```python
from build123d import *

# Parameters (mm, degrees)
SKETCH_1_R          = 27.5
SKETCH_1_R_2        = 21.5
SKETCH_1_R_3        = 1.1
EXTRUDE_1_DEPTH     = 5
CUT_EXTRUDE_1_DEPTH = 5
FILLET_1_R          = 1.5


with BuildPart() as part:
    # 草图1 → 凸台-拉伸1 (new body)
    with BuildSketch(Plane(origin=(0, 0, 0), x_dir=(1, 0, 0), z_dir=(0, 1, 0))):
        with Locations(Location((0, 0, 0), (0, 0, 270))):
            Circle(SKETCH_1_R)
        with Locations(Location((0, 0, 0), (0, 0, 270))):
            Circle(SKETCH_1_R_2, mode=Mode.SUBTRACT)
        with Locations(Location((0, 24.5, 0), (0, 0, 270))):
            Circle(SKETCH_1_R_3, mode=Mode.SUBTRACT)
        with Locations(Location((21.217622393, -12.25, 0), (0, 0, 270))):
            Circle(SKETCH_1_R_3, mode=Mode.SUBTRACT)
        with Locations(Location((-21.217622393, -12.25, 0), (0, 0, 270))):
            Circle(SKETCH_1_R_3, mode=Mode.SUBTRACT)
    extrude(amount=EXTRUDE_1_DEPTH)

    # 草图2 → 切除-拉伸1 (cut)
    with BuildSketch(Plane.XZ):
        with BuildLine():
            Line((-2.453357197, -21.359565503), (-4.550320626, -27.120925172))
            ThreePointArc((-4.550320626, -27.120925172), (-20.900792824, -17.871957345), (-27.498537849, -0.283577443))
            Line((-27.498537849, -0.283577443), (-21.481435012, 0.89328037))
            ThreePointArc((-21.481435012, 0.89328037), (-16.340619844, -13.972621197), (-2.453357197, -21.359565503))
        make_face()
    extrude(amount=-CUT_EXTRUDE_1_DEPTH, mode=Mode.SUBTRACT)

    # 圆角1
    fillet_1_edges = [part.edges().sort_by_distance(p)[0] for p in [
        (-21.481435012, 2.5, 0.89328037),
        (-2.453357197, 2.5, -21.359565503),
        (-4.550320626, 2.5, -27.120925172),
        (-27.498537849, 2.5, -0.283577443),
    ]]
    fillet(fillet_1_edges, radius=FILLET_1_R)


solid = part.part
```
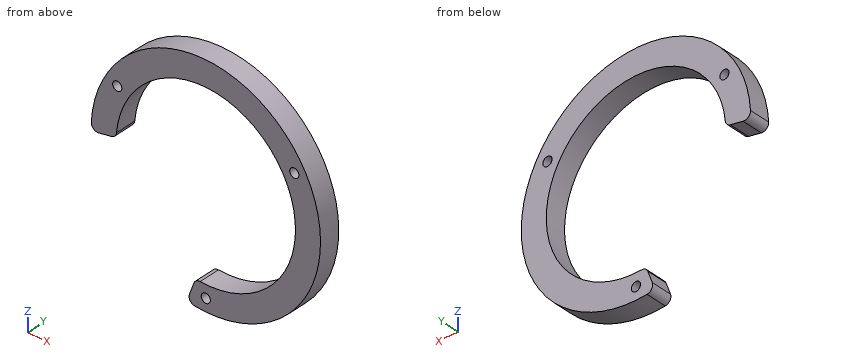
Read the model definition and answer for the solid it produces. Units are mm, in the model's axes. Coordinates: 2 decimals unless noted, no trailing zeros. Write each loop counter-clockwise with the first axis right and the second up, starting at its lowest first coordinate (ties: lowest second). Pieces come first, ordered by that corner, then holes. Notation, with made-up numbers: (72, 62.25) -> (86, 62.25) arc R16 cw to (86, 93.25) -> close; hole circle Ø2 at (57.25, 60.25). An arc over 180 degrees is marked (long way). Write item = value, one per line.
(1) Straight lines are drawn through the part: L1, parallel to X at y = 2.45, z = 12.25; L2, parallel to X at y = 4.45, z = -24.5; L3, parallel to X at y = 1.8, z = 2. For each, find the intervals that lie inside material, in ascending order. Write a range as from..to.
From the geometry:
L1 = -24.62..-22.32, -20.12..-17.67, 17.67..20.12, 22.32..24.62
L2 = -3.6..-1.1, 1.1..12.49
L3 = -27.43..-21.41, 21.41..27.43
(2) Section C-C on y = 1.85 is taken. Write down the section's boundary in (x, z), plus the area to 3 significant figures.
From the geometry:
outline = (-27.45, 1.64) arc R1.5 ccw to (-25.67, 0.07) -> (-22.61, 0.67) arc R1.5 ccw to (-21.41, 2) arc R21.5 cw (long way) to (-1.34, -21.46) arc R1.5 ccw to (-2.85, -22.44) -> (-3.91, -25.37) arc R1.5 ccw to (-2.65, -27.37) arc R27.5 ccw (long way) to start; hole circle Ø2.2 at (-21.22, 12.25); hole circle Ø2.2 at (0, -24.5); hole circle Ø2.2 at (21.22, 12.25)
area = 698 mm2
(3) Given pin 1 Ø1 at (x, y) = (10, 1.5) entering from -Z; pin 2 Ø3.5 at (x, z) = (-21.22, 12.25) entering from -Y; pin 3 Ø2 at (x, z) = (16.5, -11.5) entering from +Y; pin 4 Ø1.5 at (x, y) = (3.5, 2.5) entering from -Z, each flat-ended and moving along its own axis, determine where each tip first touches the part or whether it passes through.
From the geometry:
pin_1 = -25.81
pin_2 = 0
pin_3 = through
pin_4 = -27.36
(4) Section B-B on z = 7 is taken. Write down the section's boundary in (x, y).
From the geometry:
outline = (-26.59, 0) -> (-20.33, 0) -> (-20.33, 5) -> (-26.59, 5) -> close; (20.33, 0) -> (26.59, 0) -> (26.59, 5) -> (20.33, 5) -> close
(5) Section A-A on x = 0 is taken. Write down the section's boundary in (y, z).
From the geometry:
outline = (0, -27.5) -> (5, -27.5) -> (5, -25.6) -> (0, -25.6) -> close; (0, -23.4) -> (5, -23.4) -> (5, -21.5) -> (0, -21.5) -> close; (0, 21.5) -> (5, 21.5) -> (5, 27.5) -> (0, 27.5) -> close
(6) Section D-D on x = 17 is taken. Write down the section's boundary in (y, z), plus the area to 3 significant figures.
From the geometry:
outline = (0, -21.62) -> (5, -21.62) -> (5, -13.16) -> (0, -13.16) -> close; (0, 13.16) -> (5, 13.16) -> (5, 21.62) -> (0, 21.62) -> close
area = 84.5 mm2
